For this review, take the finished solid that the model builds, in its own axes (mm). A direction names the side the tool comes from. Give positions to 0.01 mm unless a question says otherwise; leave off trailing zeros. Write each loop counter-clockwise with the first axis right and the second up, starting at its lowest first coordinate (ties: lowest second). Pieces come first, ordered by that corner, then holes.
1) We need section D-D on z = 12.25. Give the boundary of the cut face in (x, y) (3 decimals), and give its area (3 significant figures).
2) Machinability: for faces 4 (the face through (0.058, 3.174, 6.591)), 5 (the face through (-9, 7, 14)), 6 (the face through (-5.282, 7.979, 6.512)), 7 (the face through (0, -4, 13)), 8 (the face through (5.2, 10.41, 19.07)), which of the approach directions +Z, -Z, +X, -X, +Y, -Y give a long, thin tool a straight path to every point of the face, cutting with its end or side? Answer none if there is none.
3) We need section A-A on x = 0. Give the boundary of the cut face in (y, z) (3 decimals).
4) We need section B-B on z = 17. Give the boundary of the cut face in (x, y), and give its area (3 significant figures).
5) Wall thickness on line 1 along Z through (x, y) = (-9, -7); line 2 along X through (y, z) = (2.05, 7); line 3 along Z through (x, y) = (-2, 3): over which ranges is each line inside the solid? List them lowest first.
6) Draft analysis for pull direction X (two halves, no side actions). For faces 1 (the face through (-5.125, 10.331, 19.07)), 2 (the face through (-11, 4, 9)), 3 (the face through (-10, 0.85, 9)), state which applies: pulls with the +X half, pulls with the -X half, needs draft (parallel to the pull), parting line crosses it, or undercut.
7) For P1, Ø9.5, axis at x = -11.5, y = 6, coming from the +Z side; P2, Ø2, axis at y = -5.5, z = 5, coming from the +X side; P3, Ø8.5, axis at x = 7, z = 11.5, coming from the -Y side, all flat-tipped, find the tip position at first contact; note any pin that passes through.
8) We need section C-C on y = 0. Give the boundary of the cut face in (x, z).
from build123d import *

# Parameters (mm, degrees)
SKETCH1_R               = 15
BOSS_EXTRUDE1_DEPTH     = 25
CUT_EXTRUDE1_DEPTH      = 11
SKETCH4_R               = 3.175
CUT_EXTRUDE2_DEPTH      = 14
SKETCH5_R               = 8
CUT_EXTRUDE3_DEPTH      = 1
SKETCH6_W               = 28.841933153
SKETCH6_H               = 1.7
CUT_EXTRUDE4_DEPTH      = 14
SKETCH7_W               = 7.940894739
SKETCH7_H               = 1.7
BOSS_EXTRUDE2_DEPTH     = 2
CHAMFER1_SIZE           = 11
CUT_EXTRUDE5_DEPTH      = 14
CUT_EXTRUDE5_DEPTH_BACK = 14
SKETCH8_R               = 2
SKETCH9_R               = 3.75
CUT_EXTRUDE6_DEPTH      = 11
FILLET1_R               = 2
FILLET2_R               = 1


with BuildPart() as part:
    # Sketch1 → Boss-Extrude1 (new body)
    with BuildSketch(Plane.XY):
        Circle(SKETCH1_R)
    extrude(amount=BOSS_EXTRUDE1_DEPTH)

    # Sketch3 → Cut-Extrude1 (cut)
    with BuildSketch(Plane.XY.offset(25)):
        with BuildLine():
            ThreePointArc((2.96875, -7.428763251), (31, 0), (2.96875, 7.428763251))
            ThreePointArc((2.96875, 7.428763251), (0, 8), (-2.96875, 7.428763251))
            ThreePointArc((-2.96875, 7.428763251), (-31, 0), (-2.96875, -7.428763251))
            ThreePointArc((-2.96875, -7.428763251), (0, -8), (2.96875, -7.428763251))
        make_face()
    extrude(amount=-CUT_EXTRUDE1_DEPTH, mode=Mode.SUBTRACT)

    # Sketch4 → Cut-Extrude2 (cut)
    with BuildSketch(Plane.XY.offset(14)):
        Circle(SKETCH4_R)
    extrude(amount=-CUT_EXTRUDE2_DEPTH, mode=Mode.SUBTRACT)

    # Sketch5 → Cut-Extrude3 (cut)
    with BuildSketch(Plane.XY.offset(14)):
        Circle(SKETCH5_R)
    extrude(amount=-CUT_EXTRUDE3_DEPTH, mode=Mode.SUBTRACT)

    # Sketch6 → Cut-Extrude4 (cut)
    with BuildSketch(Plane.XY.offset(14)):
        with Locations((-3.420966576, 0)):
            Rectangle(SKETCH6_W, SKETCH6_H)
    extrude(amount=-CUT_EXTRUDE4_DEPTH, mode=Mode.SUBTRACT)

    # Sketch7 → Boss-Extrude2 (add)
    with BuildSketch(Plane(origin=(0, 0, 0), x_dir=(-1, 0, 0), z_dir=(0, 0, -1))):
        with Locations((-7.02955263, 0)):
            Rectangle(SKETCH7_W, SKETCH7_H)
    extrude(amount=-BOSS_EXTRUDE2_DEPTH)

    # Chamfer1
    # the kernel refuses this chamfer: 11 mm, written as the material it adds along each edge
    with BuildSketch(Plane(origin=(11, -0.85, 2), x_dir=(0.027495876610586414, 0, 0.9996219169112968), z_dir=(0, 1, 0))) as chamfer1_piece_1_section:
        Polygon((CHAMFER1_SIZE * 0.999621916911, -CHAMFER1_SIZE * 0.0274958766106), (-CHAMFER1_SIZE * 0.0274958766106, -CHAMFER1_SIZE * 0.999621916911), (0, 0), align=None)
    chamfer1_piece_1 = extrude(amount=1.7, mode=Mode.PRIVATE)
    chamfer1_piece_1 = split(chamfer1_piece_1, bisect_by=Plane(origin=(3.059105261, 0, 5.913893193), z_dir=(1, 0, 0)), keep=Keep.TOP, mode=Mode.PRIVATE)
    add(chamfer1_piece_1)

    # Sketch8 → Cut-Extrude5 (cut, two sides: drawn at the far end of the back side and taken through both)
    with BuildSketch(Plane(origin=(0, 0, 0), x_dir=(1, 0, 0), z_dir=(0, 1, 0)).offset(-CUT_EXTRUDE5_DEPTH_BACK)):
        with Locations(Location((-9, -7, 0), (0, 0, 90))):
            Circle(SKETCH8_R)
    extrude(amount=CUT_EXTRUDE5_DEPTH + CUT_EXTRUDE5_DEPTH_BACK, mode=Mode.SUBTRACT)

    # Sketch9 → Cut-Extrude6 (cut)
    with BuildSketch(Plane(origin=(0, 15, 0), x_dir=(1, 0, 0), z_dir=(0, 1, 0))):
        with Locations(Location((-9, -7, 0), (0, 0, 270))):
            Circle(SKETCH9_R)
    extrude(amount=-CUT_EXTRUDE6_DEPTH, mode=Mode.SUBTRACT)

    # Fillet1
    fillet1_edges = [part.edges().sort_by_distance(p)[0] for p in [
        (15, 0, 0),
    ]]
    fillet(fillet1_edges, radius=FILLET1_R)

    # Fillet2
    fillet2_edges = [part.edges().sort_by_distance(p)[0] for p in [
        (-5.160499055, 10.368472369, 25),
        (0, -8, 25),
        (5.160499055, -10.368472369, 25),
        (0, 8, 25),
        (-5.160499055, -10.368472369, 25),
        (5.160499055, 10.368472369, 25),
    ]]
    fillet(fillet2_edges, radius=FILLET2_R)


solid = part.part
Results list:
1. outline: (-14.976, -0.85) arc R15 ccw (long way) to (-14.976, 0.85) - (-3.059, 0.85) arc R3.175 cw to (3.059, 0.85) - (10.25, 0.85) - (10.25, -0.85) - (3.059, -0.85) arc R3.175 cw to (-3.059, -0.85) - close
1. area: 643 mm2
2. face 4: +Z, -Z
2. face 5: +Z, -X
2. face 6: +Y
2. face 7: +Z
2. face 8: +Z, +X
3. outline: (-15, 2) arc R2 ccw to (-13, 0) - (-3.175, 0) - (-3.175, 13) - (-8, 13) - (-8, 24) arc R1 ccw to (-9, 25) - (-15, 25) - close; (3.175, 0) - (13, 0) arc R2 ccw to (15, 2) - (15, 25) - (9, 25) arc R1 ccw to (8, 24) - (8, 13) - (3.175, 13) - close
4. outline: (-8, -12.69) arc R15 ccw to (8, -12.69) arc R15 cw to (2.97, -7.43) arc R8 cw to (-2.97, -7.43) arc R15 cw to start; (-8, 12.69) arc R15 cw to (-2.97, 7.43) arc R8 cw to (2.97, 7.43) arc R15 cw to (8, 12.69) arc R15 ccw to start
4. area: 152 mm2
5. line 1: z = 0 to 5, 9 to 14
5. line 2: x = -14.86 to -11, -7 to -2.42, 2.42 to 14.86
5. line 3: z = 0 to 13
6. face 1: pulls with the -X half
6. face 2: undercut
6. face 3: needs draft
7. P1: stops at z = 14
7. P2: stops at x = 14.31
7. P3: stops at y = -14.75
8. outline: (3.06, 0) - (13, 0) arc R2 ccw to (15, 2) - (15, 14) - (11, 14) - (11, 13) - (3.06, 5.06) - close
